```python
from build123d import *

# Parameters (mm, degrees)
PAD_DEPTH    = 140
CHAMFER_SIZE = 1


with BuildPart() as part:
    # Sketch → Pad (new body, symmetric)
    with BuildSketch(Plane.XZ):
        with BuildLine():
            ThreePointArc((4.5, 0), (0, 18.505745), (-4.5, 0))
            Line((-4.5, 0), (4.5, 0))
        make_face()
    extrude(amount=PAD_DEPTH, both=True)

    # Chamfer
    chamfer_edges = [part.edges().sort_by_distance(p)[0] for p in [
        (0, -140, 18.505745),
        (0, -140, 0),
        (0, 140, 18.505745),
        (0, 140, 0),
    ]]
    chamfer(chamfer_edges, length=CHAMFER_SIZE)


solid = part.part
```
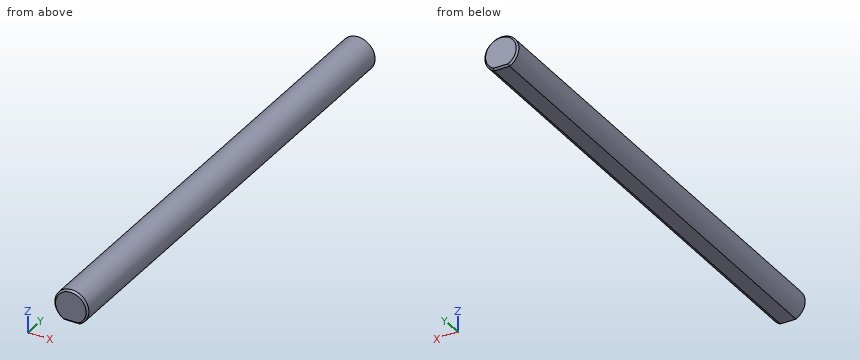
Could you check a few things on this model? Use its own coordinates, in mm. Round coordinates to 2 decimals unless told otherwise and drop trailing zeros. Loops run counter-clockwise (first coordinate to the right, second up) from the corner with the lowest first, then second, coordinate; pieces in that order, holes last. Notation, with made-up numbers: M 77,22 L 116,22 A13 cw 116,33 Z; hole C -30.5,-28.5 d2. An arc over 180 degrees is marked long. Write item = value, one per line.
1. Will these pins go through, and if not, where does the flat tip stop? P1, Ø2, axis at y = 3.5, z = 3, coming from the +X side; P2, Ø1.5, axis at y = -111.5, z = 6, coming from the +X side; P3, Ø6, axis at y = 112, z = 12, coming from the +X side.
Results below:
P1 = 8.6
P2 = 9.6
P3 = 9.8
2. I need wall thicknesses on probe 1 along X at (y, z) = (7, 8); probe 2 along Z at (x, y) = (0.5, -54); probe 3 along Z at (x, y) = (4.25, 24.5). Which ranges of each line are inside material? Lowest first, please.
Results below:
probe_1 = -9.77 to 9.77
probe_2 = 0 to 18.49
probe_3 = 0 to 17.54
3. I want a section at A-A, the plane y = 75. Write out the boundary of the cut face in (x, z).
Results below:
outline = M -4.5,0 L 4.5,0 A9.8 ccw long Z
